from build123d import *

# Parameters (mm, degrees)
SKETCH1_W                  = 25
SKETCH1_H                  = 6
SKETCH1_R                  = 0.75
BASEFRAME_DEPTH            = 2
SKETCH2_W                  = 29
SKETCH2_H                  = 6
SKETCH2_R                  = 0.75
BOSS_EXTRUDE2_DEPTH        = 2
SKETCH2_3_W                = 2
SKETCH2_3_H                = 6
BOSS_EXTRUDE3_DEPTH        = 7.1
BOSS_EXTRUDE4_DEPTH        = 6
SKETCH4_R                  = 1
SHAFTHOLE_DEPTH            = 36
SLOTBLOCK_START            = -7.1
SKETCH5_W                  = 2.5
SKETCH5_H                  = 2.5
SLOTBLOCK_DEPTH            = 5.1
SKETCH6_W                  = 0.9
SKETCH6_H                  = 0.9
SKETCH6_W_2                = 1.5
SKETCH6_H_2                = 1.5
CLIPENTRANCE_DEPTH         = 2
SKETCH6_3_W                = 0.9
SKETCH6_3_H                = 0.9
CABLEEXIT_DEPTH            = 7
SKETCH7_W                  = 1.5
SKETCH7_H                  = 1.5
CLIPLOCKSLOT_DEPTH         = 0.6
SKETCH8_W                  = 1.5
SKETCH8_H                  = 0.3
CLIPLOCKCLEARANCECUT_DEPTH = 0.5


with BuildPart() as part:
    # Sketch1 → BaseFrame (new body)
    with BuildSketch(Plane(origin=(0, 0, 0), x_dir=(1, 0, 0), z_dir=(0, 1, 0))):
        Rectangle(SKETCH1_W, SKETCH1_H)
        Circle(SKETCH1_R, mode=Mode.SUBTRACT)
    extrude(amount=BASEFRAME_DEPTH)



with BuildPart() as body_2:
    # Sketch2 → Boss-Extrude2 (new body)
    with BuildSketch(Plane(origin=(0, 7.1, 0), x_dir=(1, 0, 0), z_dir=(0, 1, 0))):
        Rectangle(SKETCH2_W, SKETCH2_H)
        Circle(SKETCH2_R, mode=Mode.SUBTRACT)
    extrude(amount=BOSS_EXTRUDE2_DEPTH)


with BuildPart() as part_1:
    add(part.part)

    add(body_2.part)  # Boss-Extrude3 merges body 2
    # Sketch2<3> → Boss-Extrude3 (add)
    with BuildSketch(Plane(origin=(0, 7.1, 0), x_dir=(1, 0, 0), z_dir=(0, 1, 0))):
        with Locations((-13.5, 0)):
            Rectangle(SKETCH2_3_W, SKETCH2_3_H)
        with Locations((13.5, 0)):
            Rectangle(SKETCH2_3_W, SKETCH2_3_H)
    extrude(amount=-BOSS_EXTRUDE3_DEPTH)

    # Sketch3 → Boss-Extrude4 (add)
    with BuildSketch(Plane(origin=(0, 0, -3), x_dir=(-1, 0, 0), z_dir=(0, 0, -1))):
        Polygon((-14.5, 9.1), (-17.5, 7.55), (-17.5, 1.55), (-14.5, 0), align=None)
        Polygon((14.5, 0), (17.5, 1.55), (17.5, 7.55), (14.5, 9.1), align=None)
    extrude(amount=-BOSS_EXTRUDE4_DEPTH)

    # Sketch4 → ShaftHole (cut, through all)
    with BuildSketch(Plane.ZY.offset(17.5)):
        with Locations((0, 4.55)):
            Circle(SKETCH4_R)
    extrude(amount=-SHAFTHOLE_DEPTH, mode=Mode.SUBTRACT)

    # Sketch5 → SlotBlock (add)
    with BuildSketch(Plane(origin=(0, 9.1, 0), x_dir=(1, 0, 0), z_dir=(0, 1, 0)).offset(SLOTBLOCK_START)):
        with Locations((7.2, -1.75)):
            Rectangle(SKETCH5_W, SKETCH5_H)
    slotblock = extrude(amount=SLOTBLOCK_DEPTH)

    # Sketch6 → ClipEntrance (cut)
    with BuildSketch(Plane.XY.offset(3)):
        with Locations((7.2, 4.55)):
            Rectangle(SKETCH6_W, SKETCH6_H)
        with Locations((7.2, 4.55)):
            Rectangle(SKETCH6_W_2, SKETCH6_H_2)
        with Locations((7.2, 4.55)):
            Rectangle(SKETCH6_W, SKETCH6_H, mode=Mode.SUBTRACT)
    clipentrance = extrude(amount=-CLIPENTRANCE_DEPTH, mode=Mode.SUBTRACT)

    # Sketch6<3> → CableExit (cut, through all)
    with BuildSketch(Plane.XY.offset(3)):
        with Locations((7.2, 4.55)):
            Rectangle(SKETCH6_3_W, SKETCH6_3_H)
    cableexit = extrude(amount=-CABLEEXIT_DEPTH, mode=Mode.SUBTRACT)

    # Sketch7 → ClipLockSlot (cut)
    with BuildSketch(Plane.XZ.offset(-5.3)):
        with Locations((7.2, 1.75)):
            Rectangle(SKETCH7_W, SKETCH7_H)
    cliplockslot = extrude(amount=-CLIPLOCKSLOT_DEPTH, mode=Mode.SUBTRACT)

    # Sketch8 → ClipLockClearanceCut (cut)
    with BuildSketch(Plane.XY.offset(3)):
        with Locations((7.2, 5.45)):
            Rectangle(SKETCH8_W, SKETCH8_H)
    cliplockclearancecut = extrude(amount=-CLIPLOCKCLEARANCECUT_DEPTH, mode=Mode.SUBTRACT)

    # Mirror1: SlotBlock, ClipEntrance, CableExit, ClipLockSlot, ClipLockClearanceCut across plane
    add(slotblock.mirror(Plane(origin=(0, 0, 0), x_dir=(0, 0, 1), z_dir=(1, 0, 0))))
    add(clipentrance.mirror(Plane(origin=(0, 0, 0), x_dir=(0, 0, 1), z_dir=(1, 0, 0))), mode=Mode.SUBTRACT)
    add(cableexit.mirror(Plane(origin=(0, 0, 0), x_dir=(0, 0, 1), z_dir=(1, 0, 0))), mode=Mode.SUBTRACT)
    add(cliplockslot.mirror(Plane(origin=(0, 0, 0), x_dir=(0, 0, 1), z_dir=(1, 0, 0))), mode=Mode.SUBTRACT)
    add(cliplockclearancecut.mirror(Plane(origin=(0, 0, 0), x_dir=(0, 0, 1), z_dir=(1, 0, 0))), mode=Mode.SUBTRACT)


solid = part_1.part
The listing builds one solid part. Answer for the finished solid, in the listing's coordinates (mm). A direction names the side the tool comes from. Give positions to 0.01 mm unless a question says otherwise; leave off trailing zeros. Write each loop counter-clockwise with the first axis right and the second up, starting at its lowest first coordinate (ties: lowest second). Pieces come first, ordered by that corner, then holes. Notation, with made-up numbers: (50, -2.75) - (98, -2.75) arc R14 cw to (98, 11.25) - close; hole circle Ø3 at (29, -40). An arc over 180 degrees is marked (long way). Use a Markdown table: item, result.
1. For a pull along Z with two mould halves and no side action, classify faces 1 (the flat face through (5.95, 5, 2)), 2 (the cylindrical face through (-0.75, 8.09, -0.03)), 3 (the flat face through (-6.6, 4.5, 0.5)), 4 (the flat face through (7, 5.9, 2)) as released by +Z, released by -Z, zero draft, split by the parting line, or undercut.
Values follow:
| item | result |
|---|---|
| face 1 | zero draft |
| face 2 | undercut |
| face 3 | released by -Z |
| face 4 | undercut |
2. Each of these flat-tipped pins is pushed along its axis until it touches: P1, Ø1.8, axis at x = -3, z = -1.5, coming from the -Y side; P2, Ø1.6, axis at y = 4.55, z = 0, coming from the -X side; P3, Ø2.5, axis at x = 7.5, y = 5.5, coming from the -Z side; P4, Ø0.8, axis at x = -7.5, y = 5, coming from the +Z side. Where does it stop, or does it pass through?
Values follow:
| item | result |
|---|---|
| P1 | stops at y = 0 |
| P2 | stops at x = -8.45 |
| P3 | stops at z = 0.5 |
| P4 | stops at z = 1 |
3. Find the intervals of material crossed by probe 1 along X at (y, z) = (2.75, 2.3); probe 2 along X at (y, z) = (5.5, 2.5); probe 3 along Z at (x, y) = (0, 8.2), in increasing order. Write a range as from..to.
Values follow:
| item | result |
|---|---|
| probe 1 | x = -17.5..-12.5, -8.45..-5.95, 5.95..8.45, 12.5..17.5 |
| probe 2 | x = -17.5..-12.5, -8.45..-7.95, -6.45..-5.95, 5.95..6.45, 7.95..8.45, 12.5..17.5 |
| probe 3 | z = -3..-0.75, 0.75..3 |
4. Section B-B on x = 0 is taken. Write down the section's boundary in (y, z).
Values follow:
| item | result |
|---|---|
| outline | (0, -3) - (2, -3) - (2, -0.75) - (0, -0.75) - close; (0, 0.75) - (2, 0.75) - (2, 3) - (0, 3) - close; (7.1, -3) - (9.1, -3) - (9.1, -0.75) - (7.1, -0.75) - close; (7.1, 0.75) - (9.1, 0.75) - (9.1, 3) - (7.1, 3) - close |
5. Section A-A on y = 2.5 is taken. Write down the section's boundary in (x, z).
Values follow:
| item | result |
|---|---|
| outline | (-17.5, -3) - (-12.5, -3) - (-12.5, 3) - (-17.5, 3) - close; (-8.45, 0.5) - (-5.95, 0.5) - (-5.95, 3) - (-8.45, 3) - close; (5.95, 0.5) - (8.45, 0.5) - (8.45, 3) - (5.95, 3) - close; (12.5, -3) - (17.5, -3) - (17.5, 3) - (12.5, 3) - close |
6. Section D-D on x = -9 is taken. Write down the section's boundary in (y, z), plus the area to 3 significant figures.
Values follow:
| item | result |
|---|---|
| outline | (0, -3) - (2, -3) - (2, 3) - (0, 3) - close; (7.1, -3) - (9.1, -3) - (9.1, 3) - (7.1, 3) - close |
| area | 24.0 mm² |
7. A tool of negligible diameter and unlimited length cuts with its end or side. For faces 5 (the flat face through (-5.95, 5, 2)), 6 (the cylindrical face through (14.97, 5.54, -0.13)), 7 (the flat face through (15.979, 8.336, -0.042)), 8 (the flat face through (-7, 5.9, 2)), from which of +Z, -Z, +X, -X, +Y, -Y can it reach the whole face along a straight path? Write none if from no direction.
Values follow:
| item | result |
|---|---|
| face 5 | +Z, -Z |
| face 6 | +X |
| face 7 | +Z, -Z, +X, +Y |
| face 8 | none |
8. Section C-C on z = 2.15 is taken. Write down the section's boundary in (x, y), plus the area to 3 significant figures.
Values follow:
| item | result |
|---|---|
| outline | (-17.5, 1.55) - (-14.5, 0) - (14.5, 0) - (17.5, 1.55) - (17.5, 7.55) - (14.5, 9.1) - (-14.5, 9.1) - (-17.5, 7.55) - close; hole (-12.5, 2) - (-8.45, 2) - (-8.45, 7.1) - (-12.5, 7.1) - close; hole (-7.95, 3.8) - (-6.45, 3.8) - (-6.45, 5.9) - (-7.95, 5.9) - close; hole (-5.95, 2) - (5.95, 2) - (5.95, 7.1) - (-5.95, 7.1) - close; hole (6.45, 3.8) - (7.95, 3.8) - (7.95, 5.9) - (6.45, 5.9) - close; hole (8.45, 2) - (12.5, 2) - (12.5, 7.1) - (8.45, 7.1) - close |
| area | 201 mm² |
